The listing builds one solid part. Answer for the finished solid, in the listing's coordinates (mm). Give positions to 0.01 mm unless a question says otherwise; leave off trailing zeros. Order: outer loops, then holes, each group sorted by start corner. A loop starts at its lowest first (then second) coordinate and runs counter-clockwise, first axis right, second up. Notation, with made-up numbers: (-25.75, 47.5) - (-6.75, 47.5) arc R15 ccw to (-6.75, 70.5) - close; hole circle Ø1 at (29.25, 31.5). An arc over 180 degrees is marked (long way). Use a Markdown table: item, result. Add a question column.
1) Flat-ended cylindrical pins translate along their axes: pin 1 (1.5 mm diameter, centred on y = -2, z = -26, fed in from -X); pin 2 (1.6 mm diameter, centred on y = -1.5, z = -8, fed in from +X); pin 3 (1.3 mm diameter, centred on y = -1.5, z = -7.5, fed in from +X). Find the tip coordinate at first contact, or state that the pin passes through.
2) Find section C-C, the plane y = -1.5. State how many separate pieces and enclosed holes the cut face has, plus the area to 3 significant figures.
3) The mould has two halves that part along X. Classify faces 1 (the face through (2.3, -1.6, -27.6)), 2 (the face through (24, -2, -23.876)): released by +X, released by -X, zero draft, split by the parting line, or undercut.
4) Find section B-B, the plane x = 25.5. Determine the outline of the cut face in (y, z) (3 decimals), plus the area to 3 significant figures.
5) Find section A-A, the plane z = -22. Determine the outline of the cut face in (x, y) (3 decimals).
6) Straight lines are drawn through the part: line 1 (X direction, y = -0.6, z = -19.5); line 2 (Z direction, x = 13, y = -0.95); line 3 (X direction, y = -1.15, z = -10). For each, find the intervals that lie inside material, in ascending order.
from build123d import *

# Parameters (mm, degrees)
F0_W     = 3.175
F0_H     = 2.972425
F1_DEPTH = 3.175


with BuildPart() as f1:
    # F0 (on Front) → F1 (new body)
    with BuildSketch(Plane.XZ):
        Polygon((38.1, 0), (0, 0), (0, -25.4), (4.699, -29.896425), (9.398, -34.595425), (47.498261, -34.595164), (47.498261, -9.195164), (42.811127, -4.508029), align=None)
        Polygon((9.398, -32.440164), (6.854261, -29.896425), (9.398, -29.896425), align=None, mode=Mode.SUBTRACT)
        Polygon((4.699, -27.787109), (2.204346, -25.4), (4.699, -25.4), align=None, mode=Mode.SUBTRACT)
        with Locations((7.8105, -26.886212)):
            Rectangle(F0_W, F0_H, mode=Mode.SUBTRACT)
        Polygon((44.898607, -33.071182), (10.922, -33.071415), (10.922, -29.896425), (41.735466, -29.896425), align=None, mode=Mode.SUBTRACT)
        Polygon((10.922, -28.372425), (10.922, -25.4), (36.982772, -25.4), (40.169899, -28.372425), align=None, mode=Mode.SUBTRACT)
        Polygon((38.1, -24.358034), (38.1, -10.719228), (41.287127, -10.719206), (41.287127, -27.330459), align=None, mode=Mode.SUBTRACT)
        Polygon((42.811127, -10.719196), (45.974261, -10.719174), (45.974261, -31.991563), (42.811127, -28.816814), align=None, mode=Mode.SUBTRACT)
        Polygon((1.524, -23.876), (1.524, -2.567819), (4.699, -5.540244), (4.699, -23.876), align=None, mode=Mode.SUBTRACT)
        Polygon((6.223, -23.876), (6.223, -7.098056), (9.398, -10.273056), (9.398, -23.876), align=None, mode=Mode.SUBTRACT)
        Polygon((10.922, -23.876), (10.922, -10.719415), (36.576, -10.719239), (36.576, -23.876), align=None, mode=Mode.SUBTRACT)
        Polygon((10.475892, -9.195418), (7.312758, -6.032029), (36.576, -6.032029), (36.576, -9.195239), align=None, mode=Mode.SUBTRACT)
        Polygon((5.826084, -4.508029), (2.638957, -1.524), (36.576, -1.524), (36.576, -4.508029), align=None, mode=Mode.SUBTRACT)
        Polygon((38.1, -6.032029), (41.287127, -6.032029), (41.287127, -9.195206), (38.1, -9.195228), align=None, mode=Mode.SUBTRACT)
        Polygon((42.811127, -9.195196), (42.811127, -6.663291), (45.343015, -9.195178), align=None, mode=Mode.SUBTRACT)
        Polygon((38.1, -4.508029), (38.1, -2.109316), (40.606781, -4.508029), align=None, mode=Mode.SUBTRACT)
    extrude(amount=F1_DEPTH)


solid = f1.part
The answers:
| question | item | result |
|---|---|---|
| 1 | pin 1 | x = 0 |
| 1 | pin 2 | x = 47.1 |
| 1 | pin 3 | x = 46.45 |
| 2 | separate pieces | 1 |
| 2 | enclosed holes | 15 |
| 2 | area | 597 mm2 |
| 3 | face 1 | released by -X |
| 3 | face 2 | undercut |
| 4 | outline | (-3.175, -34.595) - (0, -34.595) - (0, -33.071) - (-3.175, -33.071) - close; (-3.175, -29.896) - (0, -29.896) - (0, -28.372) - (-3.175, -28.372) - close; (-3.175, -25.4) - (0, -25.4) - (0, -23.876) - (-3.175, -23.876) - close; (-3.175, -10.719) - (0, -10.719) - (0, -9.195) - (-3.175, -9.195) - close; (-3.175, -6.032) - (0, -6.032) - (0, -4.508) - (-3.175, -4.508) - close; (-3.175, -1.524) - (0, -1.524) - (0, 0) - (-3.175, 0) - close |
| 4 | area | 29.0 mm2 |
| 5 | outline | (0, -3.175) - (1.524, -3.175) - (1.524, 0) - (0, 0) - close; (4.699, -3.175) - (6.223, -3.175) - (6.223, 0) - (4.699, 0) - close; (9.398, -3.175) - (10.922, -3.175) - (10.922, 0) - (9.398, 0) - close; (36.576, -3.175) - (38.1, -3.175) - (38.1, 0) - (36.576, 0) - close; (41.287, -3.175) - (42.811, -3.175) - (42.811, 0) - (41.287, 0) - close; (45.974, -3.175) - (47.498, -3.175) - (47.498, 0) - (45.974, 0) - close |
| 6 | line 1 | 0 to 1.52, 4.7 to 6.22, 9.4 to 10.92, 36.58 to 38.1, 41.29 to 42.81, 45.97 to 47.5 |
| 6 | line 2 | -34.6 to -33.07, -29.9 to -28.37, -25.4 to -23.88, -10.72 to -9.2, -6.03 to -4.51, -1.52 to 0 |
| 6 | line 3 | 0 to 1.52, 4.7 to 6.22, 9.12 to 47.5 |
